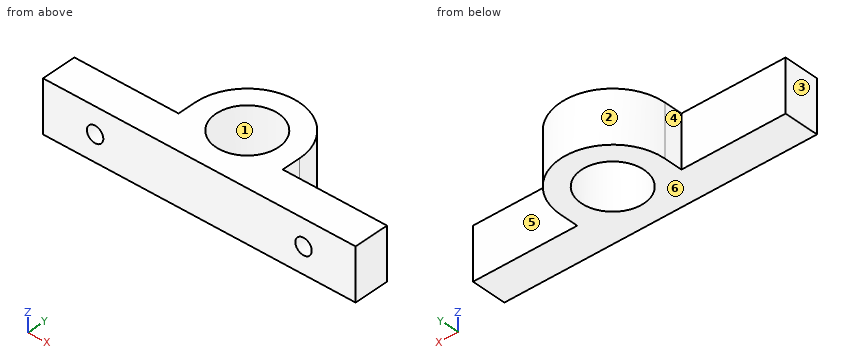
Autodesk Inventor part; units mm, degrees
ref_plane "YZ Plane" through (0, 0, 0) normal (1, 0, 0) x (0, 1, 0)
ref_plane "XZ Plane" through (0, 0, 0) normal (0, 1, 0) x (-1, 0, 0)
ref_plane "XY Plane" through (0, 0, 0) normal (0, 0, 1) x (1, 0, 0)
sketch "Sketch1" plane through (0, 0, 0) normal (0, 0, 1) x (1, 0, 0)
  line L0 (0, 0) -> (76.2, 0)
  line L1 (50.8, 8.5) -> (50.8, 13)
  line L2 (25.4, 8.5) -> (25.4, 13)
  arc A0 (50.8, 13) -> (25.4, 13) centre (38.1, 13) ccw
  line L3 (0, 8.5) -> (25.4, 8.5)
  line L4 (76.2, 8.5) -> (50.8, 8.5)
  line L5 (76.2, 8.5) -> (76.2, 0)
  line L6 (0, 8.5) -> (0, 0)
  dimension "d0" = 76.2
  dimension "d4" = 25.4
  dimension "d18" = 13
  dimension "d20" = 25.4
  dimension "d21" = 8.5
  dimension "d22" = 8.5
  dimension "d23" = 12.7
  dimension "d24" = 25.4
  dimension "d25" = 12.7
extrude "BearingBlock" add sketch "Sketch1" along normal blind 12.7
sketch "Sketch2" plane through (0, 0, 12.7) normal (0, 0, 1) x (1, 0, 0)
  arc A0 (50.8, 13) -> (25.4, 13) centre (38.1, 13) ccw
  line L0 (0, 0) -> (76.2, 0)
  circle A1 centre (38.1, 13) radius 7.62
  point P0 (38.1, 25.7)
  dimension "d8" = 15.24
  dimension "d26" = 13
extrude "BearingMount" cut sketch "Sketch2" against normal through all
sketch "Sketch3" plane through (0, 0, 0) normal (0, -1, 0) x (1, 0, 0)
  line L0 (0, 0) -> (0, 12.7)
  line L1 (-76.2, 6.35) -> (76.2, 6.35) construction
  line L2 (76.2, 0) -> (76.2, 12.7)
  circle A0 centre (12.7, 6.35) radius 2
  circle A1 centre (63.5, 6.35) radius 2
  point P0 (0, 6.35)
  dimension "d11" = 12.7
  dimension "d12" = 12.7
  dimension "d13" = 4
  dimension "d14" = 4
  dimension "d15" = 50.8
extrude "HeatSetInsert" cut sketch "Sketch3" against normal blind 7
equation "\"d18\" = motor_centerline_height"
equation "\"d13\" = m3_heat_set_insert"
equation "\"d14\" = m3_heat_set_insert"
equation "\"m3_heat_set_insert\" = 4"
equation "\"m3_clearance\" = 3.4"
equation "\"m3_heat_set_depth\" = 7"
equation "\"robot_diameter\" = 354"
equation "\"hardboard_thickness\" = 5"
equation "\"motor_centerline_height\" = 13"
properties part number "wheel_bearing2"
The listing builds one solid part. Answer for the finished solid, in the listing's coordinates (mm). Face numbers are marked on the shaded views. A direction names the side the tool comes from. Give positions to 0.01 mm unless a question says otherwise; leave off trailing zeros. Order: outer loops, then holes, each group sorted by start corner. A loop starts at its lowest first (then second) coordinate and runs counter-clockwise, first axis right, second up. Notation, with made-up numbers: (-17, 32.5) -> (-12, 32.5) arc R17 ccw to (-12, 62.5) -> close; hole circle Ø3 at (2.5, 43). An arc over 180 degrees is marked (long way). One line per item, written item: value.
1) Determine the mould class of the marked faces 1, 2 and 3 for opening direction Y: pulls with the +Y half, pulls with the -Y half, needs draft (parallel to the pull), parting line crosses it, or undercut.
Reported:
face 1: undercut
face 2: pulls with the +Y half
face 3: needs draft
2) Find section D-D, the plane x = 12.7. Determine the outline of the cut face in (y, z).
Reported:
outline: (0, 0) -> (8.5, 0) -> (8.5, 12.7) -> (0, 12.7) -> (0, 8.35) -> (7, 8.35) -> (7, 4.35) -> (0, 4.35) -> close
3) A tool of negligible diameter and unlimited length cuts with its end or side. For the marked faces 4, 5 and 6, from which of +Z, -Z, +X, -X, +Y, -Y can it reach the whole face along a straight path? Write none if from no direction.
Reported:
face 4: +Z, -Z, -X, +Y
face 5: +Z, -Z, +X, +Y
face 6: -Z, +X, -X, +Y, -Y
4) Find section B-B, the plane y = 3. Determine the outline of the cut face in (x, z), plus the area to 3 significant figures.
Reported:
outline: (0, 0) -> (76.2, 0) -> (76.2, 12.7) -> (0, 12.7) -> close; hole circle Ø4 at (12.7, 6.35); hole circle Ø4 at (63.5, 6.35)
area: 943 mm^2
5) Find section C-C, the plane y = 19.75. Determine the outline of the cut face in (x, z), plus the area to 3 significant figures.
Reported:
outline: (27.34, 0) -> (34.56, 0) -> (34.56, 12.7) -> (27.34, 12.7) -> close; (41.64, 0) -> (48.86, 0) -> (48.86, 12.7) -> (41.64, 12.7) -> close
area: 183 mm^2
6) Find section A-A, the plane z = 11.5. Determine the outline of the cut face in (x, y), plus the area to 3 significant figures.
Reported:
outline: (0, 0) -> (76.2, 0) -> (76.2, 8.5) -> (50.8, 8.5) -> (50.8, 13) arc R12.7 ccw to (25.4, 13) -> (25.4, 8.5) -> (0, 8.5) -> close; hole circle Ø15.24 at (38.1, 13)
area: 833 mm^2
7) Find the intervals of material crossed by line 1 (Z direction, x = 12.7, y = 3.5); line 2 (X direction, y = 13.5, z = 1); line 3 (Y direction, x = 38.1, z = 6), in increasing order.
Reported:
line 1: z = 0 to 4.35, 8.35 to 12.7
line 2: x = 25.41 to 30.5, 45.7 to 50.79
line 3: y = 0 to 5.38, 20.62 to 25.7
8) Flat-ended cylindrical pins translate along their axes: P1, Ø4.5, axis at x = 12.7, z = 6.35, coming from the +Y side; P2, Ø1.5, axis at y = 17.5, z = 6, coming from the +X side; P3, Ø1, axis at y = 10, z = 3.5, coming from the -X side; P4, Ø6, axis at x = 21.5, y = 19.5, coming from the +Z side. Find the tip coordinate at first contact, or state that the pin passes through.
Reported:
P1: stops at y = 8.5
P2: stops at x = 50.23
P3: stops at x = 25.4
P4: passes through
